from build123d import *

# Parameters (mm, degrees)
SKETCH1_R           = 2.665
BOSS_EXTRUDE1_DEPTH = 0.8
SKETCH2_R           = 2.335
BOSS_EXTRUDE2_DEPTH = 2.86
SKETCH3_R           = 0.23
BOSS_EXTRUDE3_DEPTH = 12.69
CIRPATTERN1_COUNT   = 3
CIRPATTERN1_ANGLE   = 180
SKETCH4_R           = 2.005
CUT_EXTRUDE1_DEPTH  = 1


with BuildPart() as part:
    # Sketch1 → Boss-Extrude1 (new body)
    with BuildSketch(Plane.XY):
        Circle(SKETCH1_R)
    extrude(amount=BOSS_EXTRUDE1_DEPTH)

    # Sketch2 → Boss-Extrude2 (add)
    with BuildSketch(Plane.XY.offset(0.8)):
        Circle(SKETCH2_R)
    extrude(amount=BOSS_EXTRUDE2_DEPTH)

    # Sketch3 → Boss-Extrude3 (add)
    with BuildSketch(Plane(origin=(0, 0, 0), x_dir=(-1, 0, 0), z_dir=(0, 0, -1))):
        with Locations(Location((0, 1.27, 0), (0, 0, 180))):
            Circle(SKETCH3_R)
    boss_extrude3 = extrude(amount=BOSS_EXTRUDE3_DEPTH)

    # CirPattern1: Boss-Extrude3 ×3 about axis
    cirpattern1_axis = Axis((0, 0, 0), (0, 0, 1))
    for i in range(1, CIRPATTERN1_COUNT):
        add(boss_extrude3.rotate(cirpattern1_axis, i * CIRPATTERN1_ANGLE / (CIRPATTERN1_COUNT - 1)))

    # Sketch4 → Cut-Extrude1 (cut)
    with BuildSketch(Plane.XY.offset(3.66)):
        Circle(SKETCH4_R)
    extrude(amount=-CUT_EXTRUDE1_DEPTH, mode=Mode.SUBTRACT)


solid = part.part
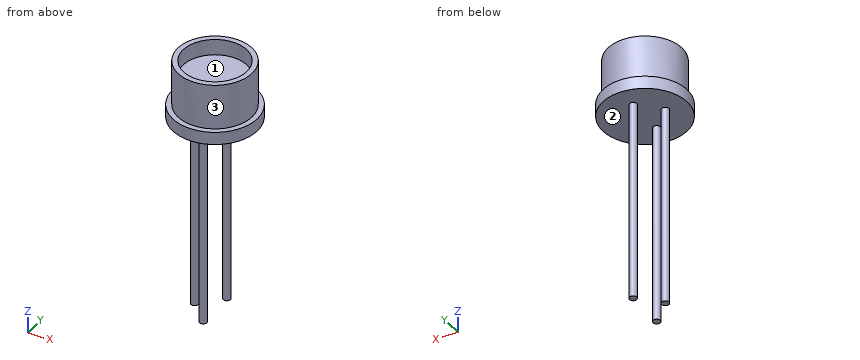
The model under review builds one solid part; all positions refer to its coordinate system, in mm. Face numbers are marked on the shaded views. Round coordinates to 2 decimals unless told otherwise and drop trailing zeros. Order: outer loops, then holes, each group sorted by start corner. A loop starts at its lowest first (then second) coordinate and runs counter-clockwise, first axis right, second up. Notation, with made-up numbers: (71, -33.5) -> (94, -33.5) arc R25 ccw to (94, -18.5) -> close; hole circle Ø1 at (54, -13.75). An arc over 180 degrees is marked (long way). Write item = value, one per line. Start each with the question number.
Item 1: Consider section C-C on z = -3. Write out the cut boundary in (x, y).
Item 2: Mouldability with a two-part tool opening along X and no side actions: class the marked faces 1, 2 and 3 as released by +X, released by -X, zero draft, split by the parting line, or undercut.
Item 3: Consider section B-B on x = 0. Write out the cut boundary in (y, z) (3 decimals), plus the area to 3 significant figures.
Item 4: Clearance check with flat-ended pins moving along their axes: pin 1 Ø2.5 at (x, y) = (0.5, 1) entering from -Z; pin 2 Ø1.2 at (x, y) = (-0.5, -1) entering from +Z. State where each tip first meets the part, or that it passes through.
Item 5: For line 1 along Y through (x, z) = (0, 3.35) (3 decimals); line 2 along Z through (x, y) = (0.15, 1.6); line 3 along Z through (x, y) = (1.15, 2.3), list the stretches that pass through material, from the lowest coordinate up.
Item 6: Consider section D-D on z = 2.25. Write out the cut boundary in (x, y) (3 decimals), plus the area to 3 significant figures.
Item 7: Consider section A-A on y = 0. Write out the cut boundary in (x, z) (3 decimals).
Conclusion:
q1.outline = circle Ø0.46 at (-1.27, 0); circle Ø0.46 at (0, -1.27); circle Ø0.46 at (0, 1.27)
q2.face_1 = undercut
q2.face_2 = zero draft
q2.face_3 = split by the parting line
q3.outline = (-2.665, 0) -> (-1.5, 0) -> (-1.5, -12.69) -> (-1.04, -12.69) -> (-1.04, 0) -> (1.04, 0) -> (1.04, -12.69) -> (1.5, -12.69) -> (1.5, 0) -> (2.665, 0) -> (2.665, 0.8) -> (2.335, 0.8) -> (2.335, 3.66) -> (2.005, 3.66) -> (2.005, 2.66) -> (-2.005, 2.66) -> (-2.005, 3.66) -> (-2.335, 3.66) -> (-2.335, 0.8) -> (-2.665, 0.8) -> close
q3.area = 25.3 mm2
q4.pin_1 = -12.69
q4.pin_2 = 2.66
q5.line_1 = -2.335 to -2.005, 2.005 to 2.335
q5.line_2 = 0 to 2.66
q5.line_3 = 0 to 0.8
q6.outline = circle Ø4.67 at (0, 0)
q6.area = 17.1 mm2
q7.outline = (-2.665, 0) -> (-1.5, 0) -> (-1.5, -12.69) -> (-1.04, -12.69) -> (-1.04, 0) -> (2.665, 0) -> (2.665, 0.8) -> (2.335, 0.8) -> (2.335, 3.66) -> (2.005, 3.66) -> (2.005, 2.66) -> (-2.005, 2.66) -> (-2.005, 3.66) -> (-2.335, 3.66) -> (-2.335, 0.8) -> (-2.665, 0.8) -> close
